Design review of the part built by this model. Coordinates are the model's own, in mm. Face numbers are marked on the shaded views. A direction names the side the tool comes from. Give positions to 0.01 mm unless a question says otherwise; leave off trailing zeros. Write each loop counter-clockwise with the first axis right and the second up, starting at its lowest first coordinate (ties: lowest second). Pieces come first, ordered by that corner, then holes. Notation, with made-up numbers: M -37,-15 L 11,-15 A26 cw 11,5 Z; hole C -33.5,39 d9. An arc over 180 degrees is marked long. One line per item, written item: value. Start each with the question number.
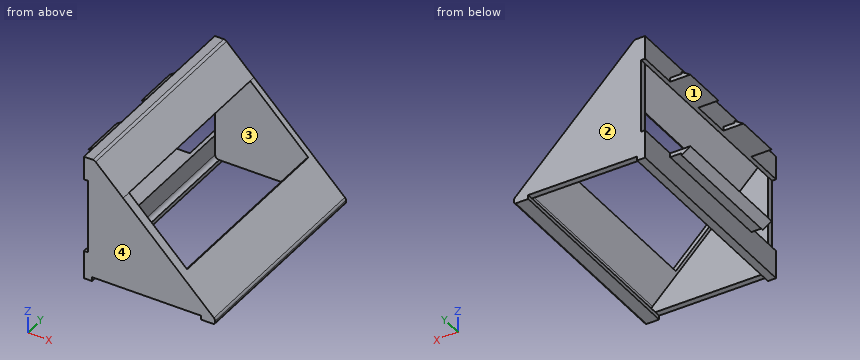
```python
from build123d import *

# Parameters (mm, degrees)
F1_DEPTH      = 3
F1_DEPTH_BACK = 101.7
F2_DEPTH      = 98.7
F3_DEPTH      = 97
F4_W          = 10
F4_H          = 0.3
F4_H_2        = 20
F4_H_3        = 19.7
F5_DEPTH      = 25
F6_W          = 10
F6_H          = 20
F6_H_2        = 19.7
F7_DEPTH      = 50


with BuildPart() as f1:
    # F0 (on Front) → F1 (new body, two sides)
    with BuildSketch(Plane.XZ) as f1_sk:
        with BuildLine():
            Line((0, 52.7286796564), (0, 50.7286796564))
            Line((0, 50.7286796564), (2, 50.7286796564))
            Line((2, 50.7286796564), (2, 57.9289321881))
            ThreePointArc((2, 57.9289321881), (3.2346331353, 59.7766912532), (5.4142135624, 59.3431457505))
            Line((5.4142135624, 59.3431457505), (17.9890566593, 46.7683026536))
            Line((17.9890566593, 46.7683026536), (19.4032702217, 48.182516216))
            Line((19.4032702217, 48.182516216), (5.7928932188, 61.7928932188))
            ThreePointArc((5.7928932188, 61.7928932188), (5.1440465212, 62.2264387215), (4.3786796564, 62.3786796564))
            Line((4.3786796564, 62.3786796564), (0, 62.3786796564))
            Line((0, 62.3786796564), (0, 52.7286796564))
        make_face()
        with BuildLine():
            ThreePointArc((2, 4), (2.5857864376, 2.5857864376), (4, 2))
            Line((4, 2), (57.9289321881, 2))
            ThreePointArc((57.9289321881, 2), (59.7766912532, 3.2346331353), (59.3431457505, 5.4142135624))
            Line((59.3431457505, 5.4142135624), (46.7683026536, 17.9890566593))
            Line((46.7683026536, 17.9890566593), (17.9890566593, 46.7683026536))
            Line((17.9890566593, 46.7683026536), (5.4142135624, 59.3431457505))
            ThreePointArc((5.4142135624, 59.3431457505), (3.2346331353, 59.7766912532), (2, 57.9289321881))
            Line((2, 57.9289321881), (2, 50.7286796564))
            Line((2, 50.7286796564), (2, 14.0286796564))
            Line((2, 14.0286796564), (2, 4))
        make_face()
        with BuildLine():
            Line((57.9289321881, 2), (57.9289321881, 0))
            Line((57.9289321881, 0), (64, 0))
            ThreePointArc((64, 0), (64.7071067812, 0.2928932188), (65, 1))
            Line((65, 1), (65, 1.7573593129))
            ThreePointArc((65, 1.7573593129), (64.847759065, 2.5227261776), (64.4142135624, 3.1715728753))
            Line((64.4142135624, 3.1715728753), (48.182516216, 19.4032702217))
            Line((48.182516216, 19.4032702217), (46.7683026536, 17.9890566593))
            Line((46.7683026536, 17.9890566593), (59.3431457505, 5.4142135624))
            ThreePointArc((59.3431457505, 5.4142135624), (59.7766912532, 3.2346331353), (57.9289321881, 2))
        make_face()
        Polygon((-5.6, 12.0286796564), (0, 12.0286796564), (0, 14.0286796564), (-10, 14.0286796564), (-5.6, 11.0286796564), align=None)
        Polygon((-10, 50.7286796564), (0, 50.7286796564), (0, 52.7286796564), (-5.6, 52.7286796564), (-5.6, 53.7286796564), align=None)
        Polygon((17.9890566593, 46.7683026536), (46.7683026536, 17.9890566593), (48.182516216, 19.4032702217), (19.4032702217, 48.182516216), align=None)
        with BuildLine():
            Line((0, 12.0286796564), (0, 0))
            Line((0, 0), (4, 0))
            Line((4, 0), (4, 2))
            ThreePointArc((4, 2), (2.5857864376, 2.5857864376), (2, 4))
            Line((2, 4), (2, 14.0286796564))
            Line((2, 14.0286796564), (0, 14.0286796564))
            Line((0, 14.0286796564), (0, 12.0286796564))
        make_face()
    extrude(amount=-F1_DEPTH)
    extrude(f1_sk.sketch, amount=F1_DEPTH_BACK)

    # F0 (on Front) → F2 (cut)
    with BuildSketch(Plane.XZ):
        with BuildLine():
            ThreePointArc((2, 4), (2.5857864376, 2.5857864376), (4, 2))
            Line((4, 2), (57.9289321881, 2))
            ThreePointArc((57.9289321881, 2), (59.7766912532, 3.2346331353), (59.3431457505, 5.4142135624))
            Line((59.3431457505, 5.4142135624), (46.7683026536, 17.9890566593))
            Line((46.7683026536, 17.9890566593), (17.9890566593, 46.7683026536))
            Line((17.9890566593, 46.7683026536), (5.4142135624, 59.3431457505))
            ThreePointArc((5.4142135624, 59.3431457505), (3.2346331353, 59.7766912532), (2, 57.9289321881))
            Line((2, 57.9289321881), (2, 50.7286796564))
            Line((2, 50.7286796564), (2, 14.0286796564))
            Line((2, 14.0286796564), (2, 4))
        make_face()
    extrude(amount=F2_DEPTH, mode=Mode.SUBTRACT)

    # F0 (on Front) → F3 (cut)
    with BuildSketch(Plane.XZ):
        Polygon((17.9890566593, 46.7683026536), (46.7683026536, 17.9890566593), (48.182516216, 19.4032702217), (19.4032702217, 48.182516216), align=None)
    extrude(amount=F3_DEPTH, mode=Mode.SUBTRACT)

    # F4 (on face) → F5 (cut)
    with BuildSketch(Plane(origin=(0, 0, 50.7286796564), x_dir=(1, 0, 0), z_dir=(0, 0, -1))):
        with Locations((-5, 101.85)):
            Rectangle(F4_W, F4_H)
        Polygon((-10, 49.5), (-10, 39.5), (0, 39.5), (0, 49.5), (0, 59.5), (-10, 59.5), align=None)
        with Locations((-5, 7)):
            Rectangle(F4_W, F4_H_2)
        with Locations((-5, 91.85)):
            Rectangle(F4_W, F4_H_3)
    extrude(amount=-F5_DEPTH, mode=Mode.SUBTRACT)

    # F6 (on face) → F7 (cut)
    with BuildSketch(Plane(origin=(0, 0, 50.7286796564), x_dir=(1, 0, 0), z_dir=(0, 0, -1))):
        with Locations((-5, 7)):
            Rectangle(F6_W, F6_H)
        with Locations((-5, 91.85)):
            Rectangle(F6_W, F6_H_2)
    extrude(amount=F7_DEPTH, mode=Mode.SUBTRACT)


solid = f1.part
```
Q1. Machinability: for the marked faces 1 and 2, which of the approach directions +Z, -Z, +X, -X, +Y, -Y give a long, thin tool a straight path to every point of the face, cutting with its end or side? Answer none if there is none.
Q2. Take a section at A-A, the plane y = -73. State how many separate pieces and enclosed holes the cut face has, then the cut area to 3 significant figures.
Q3. Take a section at D-D, the plane x = 51.5. Give the boundary of the cut face in (y, z).
Q4. Wall thickness on line 1 (Y direction, x = 30.5, z = 4.5); line 2 (Z direction, x = 1.5, y = -68); line 3 (Y direction, x = 41.5, z = 25.5): over which ranges is each line inside the solid? List them lowest first. Write a range as from..to.
Q5. Take a section at B-B, the plane x = 28. Give the boundary of the cut face in (y, z), then the cut area to 3 significant figures.
Q6. For P1, Ø4, axis at y = -50, z = 55.5, coming from the +X side; P2, Ø5, axis at y = -27.5, z = 9.5, coming from the +X side; P3, Ø2.5, axis at x = -5.5, z = 52, coming from the +Y side, all flat-tipped, find the tip position at first contact; note any pin that passes through.
Q7. The part is to be moulded in two halves that separate along X. For the marked faces 3 and 4, say which applies: pulls with the +X half, pulls with the -X half, needs draft (parallel to the pull), parting line crosses it, or undercut.
Q8. Take a section at C-C, the plane z = 43. Give the boundary of the cut face in (x, y).
Results list:
1. face 1: -X, +Y, -Y
1. face 2: +Z, -Z, +X, -X, +Y
2. separate pieces: 3
2. enclosed holes: 0
2. area: 205 mm^2
3. outline: M -101.7,2 L -98.7,2 L -98.7,13.26 L 0,13.26 L 0,2 L 3,2 L 3,16.09 L -101.7,16.09 Z
4. line 1: y = -101.7..-98.7, 0..3
4. line 2: z = 0..14.03, 50.73..62.38
4. line 3: y = -101.7..-97, 0..3
5. outline: M -101.7,2 L -98.7,2 L -98.7,36.76 L -97,36.76 L -97,39.59 L -101.7,39.59 Z; M 0,2 L 3,2 L 3,39.59 L 0,39.59 Z
5. area: 230 mm^2
6. P1: stops at x = 14.09
6. P2: stops at x = 60.59
6. P3: stops at y = -17
7. face 3: undercut
7. face 4: needs draft
8. outline: M 2,-101.7 L 24.59,-101.7 L 24.59,-97 L 21.76,-97 L 21.76,-98.7 L 2,-98.7 Z; M 2,0 L 24.59,0 L 24.59,3 L 2,3 Z
